Geometry check sheet. Reference: the model listing, model coordinates, mm. Face numbers are marked on the shaded views. A direction names the side the tool comes from. Round coordinates to 2 decimals unless told otherwise and drop trailing zeros. Write each loop counter-clockwise with the first axis right and the second up, starting at its lowest first coordinate (ties: lowest second). Pieces come first, ordered by that corner, then holes. Notation, with made-up numbers: M 27.5,31.5 L 31.5,31.5 A11 cw 31.5,35.5 Z; hole C -13.5,38.5 d3. An arc over 180 degrees is marked long. Put each result on its own line as item: value. Start each with the question number.
(1) Section check C-C on z = 2.75. Count the separate pieces of the cut face and the enclosed holes in it, then the cut area to 3 significant figures.
(2) Tool access check on the marked faces 1 and 2. Record the directions out of +Z, -Z, +X, -X, +Y, -Y that give a thin tool (end or side, any length) a straight path to the whole face; none if there is none.
(3) Section check B-B on y = 2. Record the cut outline in (x, z).
(4) Material ranges on probe 1 along X at (y, z) = (-1.4, 0) (1 decimal); probe 2 along Y at (x, z) = (-2, -8.75); probe 3 along Z at (x, y) = (-25, 2.75), recorded low to high.
(5) Gauge pin test, flat ends, axial feed: pin 1 (5 mm diameter, centred on x = -1.5, z = 3, fed in from +Y); pin 2 (5 mm diameter, centred on x = -2.5, y = 9.5, fed in from +Z). Record the tip position at first contact, or that the pin passes through.
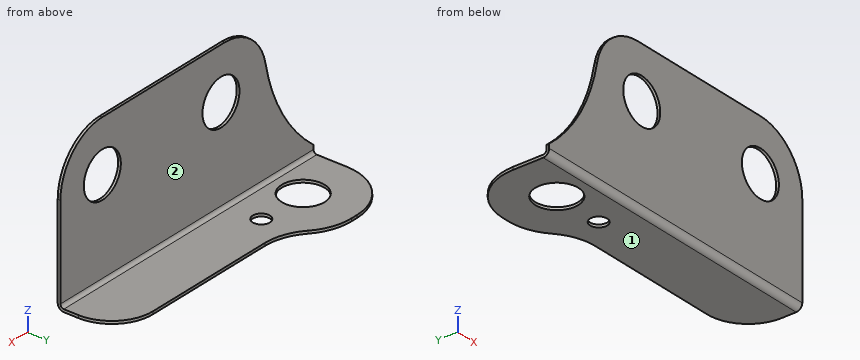
from build123d import *

# Parameters (mm, degrees)
SKETCH1_R                    = 3.3655
BOSS_EXTRUDE1_DEPTH          = 1.524
SKETCH2_R                    = 3.3655
CUT_EXTRUDE1_DEPTH           = 1.524
CUT_EXTRUDE1_DRAFT           = 46
CUT_EXTRUDE1_PROFILE_2_DEPTH = 1.524
CUT_EXTRUDE1_PROFILE_2_DRAFT = 46
FILLET1_R                    = 25.4
SKETCH3_W                    = 15.875
SKETCH3_H                    = 1.524
BOSS_EXTRUDE2_DEPTH          = 11.7475
FILLET3_R                    = 7.9375
SKETCH5_W                    = 30.1625
SKETCH5_H                    = 1.524
BOSS_EXTRUDE3_DEPTH          = 7.62
SKETCH4_R                    = 3.175
SKETCH4_R_2                  = 1.27
CUT_EXTRUDE2_DEPTH           = 19.05
FILLET7_R                    = 7.62
FILLET10_R                   = 6.096
FILLET13_R                   = 7.9375
FILLET14_R                   = 7.9375
CONVERT_SOLID1_START         = -0.62672976
CONVERT_SOLID1_OUTLINE_R     = 3.3655
CONVERT_SOLID1_DEPTH         = 12.37422976
CONVERT_SOLID1_START_2       = -1.124
CONVERT_SOLID1_2_OUTLINE_R   = 3.3655
CONVERT_SOLID1_2_DEPTH       = 0.508
CONVERT_SOLID1_START_3       = -1.524
CONVERT_SOLID1_3_OUTLINE_R   = 3.3655
CONVERT_SOLID1_3_DEPTH       = 0.4
CONVERT_SOLID1_START_4       = -27.6225
CONVERT_SOLID1_4_DEPTH       = 46.0375


with BuildPart() as part:
    # Sketch1 → Boss-Extrude1 (new body)
    with BuildSketch(Plane(origin=(0, 0, 0), x_dir=(1, 0, 0), z_dir=(0, 1, 0))):
        Polygon((-27.6225, 14.6328892), (-27.6225, 13.1088892), (-18.415, 6.7588892), (-18.415, -7.62), (18.415, -7.62), (18.415, 14.6328892), align=None)
        with Locations(Location((-10.795, 0, 0), (0, 0, 270))):
            Circle(SKETCH1_R, mode=Mode.SUBTRACT)
        with Locations(Location((10.795, 0, 0), (0, 0, 270))):
            Circle(SKETCH1_R, mode=Mode.SUBTRACT)
    extrude(amount=-BOSS_EXTRUDE1_DEPTH)


with BuildPart() as cut_extrude1_tool:
    # Sketch2 → Cut-Extrude1 (with draft: the straight prism first)
    with BuildSketch(Plane.XZ.offset(1.524)):
        with Locations((-10.795, 0)):
            Circle(SKETCH2_R)
    extrude(amount=-CUT_EXTRUDE1_DEPTH)
    # Cut-Extrude1: the draft: its side faces are tilted about the plane it starts from
    cut_extrude1_sides = [cut_extrude1_tool.faces().sort_by_distance(p)[0] for p in [
        (-14.1605, -0.762, 0),
    ]]
    draft(cut_extrude1_sides, Plane.XZ.offset(1.524), CUT_EXTRUDE1_DRAFT)


with BuildPart() as part_1:
    add(part.part)

    # Cut-Extrude1: cut by cut_extrude1_tool
    add(cut_extrude1_tool.part, mode=Mode.SUBTRACT)


with BuildPart() as cut_extrude1_profile_2_tool:
    # Sketch2 → Cut-Extrude1 profile 2 (with draft: the straight prism first)
    with BuildSketch(Plane.XZ.offset(1.524)):
        with Locations((10.795, 0)):
            Circle(SKETCH2_R)
    extrude(amount=-CUT_EXTRUDE1_PROFILE_2_DEPTH)
    # Cut-Extrude1 profile 2: the draft: its side faces are tilted about the plane it starts from
    cut_extrude1_profile_2_sides = [cut_extrude1_profile_2_tool.faces().sort_by_distance(p)[0] for p in [
        (7.4295, -0.762, 0),
    ]]
    draft(cut_extrude1_profile_2_sides, Plane.XZ.offset(1.524), CUT_EXTRUDE1_PROFILE_2_DRAFT)


with BuildPart() as part_2:
    add(part_1.part)

    # Cut-Extrude1 profile 2: cut by cut_extrude1_profile_2_tool
    add(cut_extrude1_profile_2_tool.part, mode=Mode.SUBTRACT)

    # Fillet1
    # the kernel refuses this fillet: 25.4 mm, written as the material it adds along each edge
    with BuildSketch(Plane(origin=(-18.415, 0, -6.7588892), x_dir=(0, 0, 1), z_dir=(0, -1, 0))) as fillet1_piece_1:
        with BuildLine():
            CenterArc((13.219439025, 25.4), FILLET1_R, 219.605652394, 50.394347606)
            Line((-6.35, 9.2075), (-6.74138878, 8.88365))
            ThreePointArc((-6.74138878, 8.88365), (-3.593192095, 4.315341658), (-0.418192095, -0.288408342))
            Line((-0.418192095, -0.288408342), (0, -0.508))
            Line((0, -0.508), (13.219439025, -0.508))
            Line((13.219439025, -0.508), (13.219439025, 0))
        make_face()
    extrude(amount=1.524)

    # Sketch3 → Boss-Extrude2 (add)
    with BuildSketch(Plane(origin=(0, 0, 0), x_dir=(1, 0, 0), z_dir=(0, 1, 0))):
        with Locations((-19.685, 13.8708892)):
            Rectangle(SKETCH3_W, SKETCH3_H)
    extrude(amount=BOSS_EXTRUDE2_DEPTH)

    # Fillet3
    fillet3_edges = [part_2.edges().sort_by_distance(p)[0] for p in [
        (-27.6225, 11.7475, -13.8708892),
    ]]
    fillet(fillet3_edges, radius=FILLET3_R)

    # Sketch5 → Boss-Extrude3 (add)
    with BuildSketch(Plane(origin=(0, 0, 0), x_dir=(1, 0, 0), z_dir=(0, 1, 0))):
        with Locations((3.33375, 13.8708892)):
            Rectangle(SKETCH5_W, SKETCH5_H)
    extrude(amount=BOSS_EXTRUDE3_DEPTH)

    # Sketch4 → Cut-Extrude2 (cut)
    with BuildSketch(Plane.XY.offset(-13.1088892)):
        with Locations((-19.685, 3.81)):
            Circle(SKETCH4_R)
        with Locations((-12.065, 3.81)):
            Circle(SKETCH4_R_2)
    extrude(amount=-CUT_EXTRUDE2_DEPTH, mode=Mode.SUBTRACT)

    # Fillet7
    fillet7_edges = [part_2.edges().sort_by_distance(p)[0] for p in [
        (18.415, -0.762, 7.62),
        (-18.415, -0.762, 7.62),
    ]]
    fillet(fillet7_edges, radius=FILLET7_R)

    # Fillet10
    fillet10_edges = [part_2.edges().sort_by_distance(p)[0] for p in [
        (18.415, 7.62, -13.8708892),
    ]]
    fillet(fillet10_edges, radius=FILLET10_R)

    # Fillet13
    # the kernel refuses this fillet: 7.9375 mm, written as the material it takes off along each edge
    with BuildSketch(Plane(origin=(-11.7475, 11.7475, -32.041185758), x_dir=(0, -1, 0), z_dir=(0, 0, 1))) as fillet13_piece_1:
        with BuildLine():
            CenterArc((7.9375, -6.963318623), FILLET13_R, 118.685402014, 61.314597986)
            Line((0, -6.963318623), (-0.15875, -6.963318623))
            Line((-0.15875, -6.963318623), (-0.15875, 0))
            Line((-0.15875, 0), (0, 0.15875))
            ThreePointArc((0, 0.15875), (2.06375, 0.15875), (4.0513, 0.139266372))
            Line((4.0513, 0.139266372), (4.1275, 0))
        make_face()
    extrude(amount=36.340593117, mode=Mode.SUBTRACT)

    # Fillet14
    fillet14_edges = [part_2.edges().sort_by_distance(p)[0] for p in [
        (-11.7475, 7.62, -13.8708892),
    ]]
    fillet(fillet14_edges, radius=FILLET14_R)

    # Convert-Solid1: read off the stored shape, not the designer's step
    # Convert-Solid1 outline → Convert-Solid1 (cut)
    with BuildSketch(Plane(origin=(0, 0, 0), x_dir=(1, 0, 0), z_dir=(0, 1, 0)).offset(CONVERT_SOLID1_START)):
        with BuildLine():
            Line((18.415, 14.2328892), (-27.6225, 14.2328892))
            Line((-27.6225, 14.2328892), (-27.6225, 13.1088892))
            ThreePointArc((-27.6225, 13.1088892), (-22.006205533, 6.560067822), (-18.905914469, -1.490896113))
            ThreePointArc((-18.905914469, -1.490896113), (-16.265567707, -5.891732699), (-11.43318881, -7.62))
            Line((-11.43318881, -7.62), (10.795, -7.62))
            ThreePointArc((10.795, -7.62), (16.183153673, -5.388153673), (18.415, 0))
            Line((18.415, 0), (18.415, 14.2328892))
        make_face()
        with Locations((10.795, 0)):
            Circle(CONVERT_SOLID1_OUTLINE_R, mode=Mode.SUBTRACT)
        with Locations((-10.795, 0)):
            Circle(CONVERT_SOLID1_OUTLINE_R, mode=Mode.SUBTRACT)
    extrude(amount=CONVERT_SOLID1_DEPTH, mode=Mode.SUBTRACT)

    # Convert-Solid1 2 outline → Convert-Solid1 2 (cut)
    with BuildSketch(Plane(origin=(0, 0, 0), x_dir=(1, 0, 0), z_dir=(0, 1, 0)).offset(CONVERT_SOLID1_START_2)):
        with BuildLine():
            Line((18.415, 0), (18.415, 13.1088892))
            Line((18.415, 13.1088892), (-27.6225, 13.1088892))
            ThreePointArc((-27.6225, 13.1088892), (-22.006205533, 6.560067822), (-18.905914469, -1.490896113))
            ThreePointArc((-18.905914469, -1.490896113), (-16.265567707, -5.891732699), (-11.43318881, -7.62))
            Line((-11.43318881, -7.62), (10.795, -7.62))
            ThreePointArc((10.795, -7.62), (16.183153673, -5.388153673), (18.415, 0))
        make_face()
        with Locations((-10.795, 0)):
            Circle(CONVERT_SOLID1_2_OUTLINE_R, mode=Mode.SUBTRACT)
        with Locations((10.795, 0)):
            Circle(CONVERT_SOLID1_2_OUTLINE_R, mode=Mode.SUBTRACT)
    extrude(amount=CONVERT_SOLID1_2_DEPTH, mode=Mode.SUBTRACT)

    # Convert-Solid1 3 outline → Convert-Solid1 3 (add)
    with BuildSketch(Plane(origin=(0, 0, 0), x_dir=(1, 0, 0), z_dir=(0, 1, 0)).offset(CONVERT_SOLID1_START_3)):
        with BuildLine():
            Line((18.415, 0), (18.415, 13.1088892))
            Line((18.415, 13.1088892), (-27.6225, 13.1088892))
            ThreePointArc((-27.6225, 13.1088892), (-22.006205533, 6.560067822), (-18.905914469, -1.490896113))
            ThreePointArc((-18.905914469, -1.490896113), (-16.265567707, -5.891732699), (-11.43318881, -7.62))
            Line((-11.43318881, -7.62), (10.795, -7.62))
            ThreePointArc((10.795, -7.62), (16.183153673, -5.388153673), (18.415, 0))
        make_face()
        with Locations((-10.795, 0)):
            Circle(CONVERT_SOLID1_3_OUTLINE_R, mode=Mode.SUBTRACT)
        with Locations((10.795, 0)):
            Circle(CONVERT_SOLID1_3_OUTLINE_R, mode=Mode.SUBTRACT)
    extrude(amount=CONVERT_SOLID1_3_DEPTH)

    # Convert-Solid1 4 outline → Convert-Solid1 4 (cut)
    with BuildSketch(Plane.YZ.offset(CONVERT_SOLID1_START_4)):
        with BuildLine():
            ThreePointArc((-0.62672976, -14.632825801), (-1.261835359, -14.36313734), (-1.524, -13.7248892))
            Line((-1.524, -13.7248892), (-1.524000001, -13.1088892))
            Line((-1.524000001, -13.1088892), (-3, -13.1088892))
            Line((-3, -13.1088892), (-3, -16))
            Line((-3, -16), (-0.62672976, -16))
            Line((-0.62672976, -16), (-0.62672976, -14.632825801))
        make_face()
        with BuildLine():
            Line((-0.62672976, -13.1088892), (-1.124, -13.1088892))
            Line((-1.124, -13.1088892), (-1.124, -13.7248892))
            ThreePointArc((-1.124, -13.7248892), (-0.978983965, -14.080285656), (-0.62672976, -14.232775873))
            Line((-0.62672976, -14.232775873), (-0.62672976, -13.1088892))
        make_face()
    extrude(amount=CONVERT_SOLID1_4_DEPTH, mode=Mode.SUBTRACT)


solid = part_2.part
Answers follow:
1. separate pieces: 3
1. enclosed holes: 0
1. area: 11.5 mm^2
2. face 1: -Z, +X, -X, +Y, -Y
2. face 2: +Z, +X, -X, +Y
3. outline: M -27.62,-14.63 L -22.29,-14.63 L -22.29,-14.23 L -27.62,-14.23 Z; M -17.08,-14.63 L 18.4,-14.63 L 18.4,-14.23 L -17.08,-14.23 Z
4. probe 1: x = -19.3 to -14.2, -7.4 to 7.4, 14.2 to 18.4
4. probe 2: y = -1.52 to -1.12
4. probe 3: z = -14.63 to -14.23
5. pin 1: stops at y = -1.12
5. pin 2: stops at z = -14.23
